Geometry check sheet. Reference: the model listing, model coordinates, mm. Face numbers are marked on the shaded views. Coordinates: 2 decimals unless noted, no trailing zeros. Loops run counter-clockwise (first coordinate to the right, second up) from the corner with the lowest first, then second, coordinate; pieces in that order, holes last. Notation, with made-up numbers: (51.25, 33) - (82.25, 33) arc R17 ccw to (82.25, 58) - close; hole circle Ø9 at (43, -14.75). An arc over 180 degrees is marked (long way). Write item = value, one per line. Start each with the question number.
from build123d import *

# Parameters (mm, degrees)
F0_W     = 200
F0_H     = 100
F1_DEPTH = 220
F2_T     = -12


with BuildPart() as f1:
    # F0 (on Front) → F1 (new body)
    with BuildSketch(Plane.XZ):
        Rectangle(F0_W, F0_H)
    extrude(amount=-F1_DEPTH)

    # F2
    f2_openings = [f1.faces().sort_by_distance(p)[0] for p in [
        (0, 0, 0),
    ]]
    offset(amount=F2_T, openings=f2_openings)


solid = f1.part
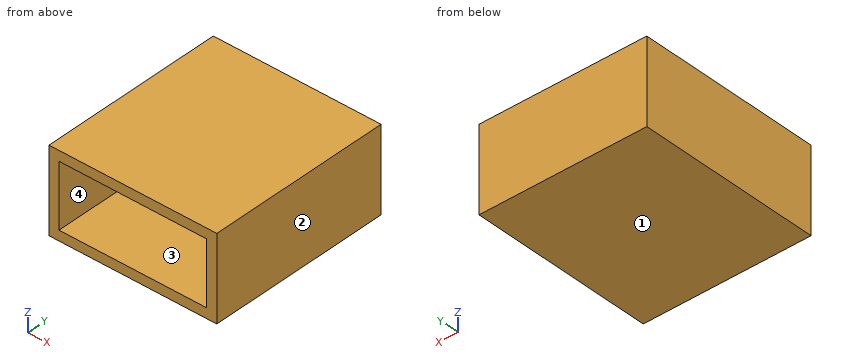
(1) Sectioned sample at C-C on y = 66. Enter the section's corners in (x, z).
(2) Depth check by flat-ended pin: pin 1 (12 mm diameter, centred on x = 73, z = 12, fed in from -Y). Enter the tip coordinate at first touch or a pass-through.
(3) Sectioned sample at A-A on x = -78. Enter the section's corners in (y, z).
(4) Scan lines: line 1 (X direction, y = 21, z = 15); line 2 (Z direction, x = -10.5, y = 177); line 3 (Y direction, x = 74, z = -29). Record each from-to range of solid material in increasing order.
(5) Sectioned sample at B-B on z = -30. Enter the section's corners in (x, y).
(6) Draft check along Z on the marked faces 1, 2, 3 and 4. Enter one of: pulls with the +Z half, pulls with the -Z half, needs draft (parallel to the pull), parting line crosses it, or undercut.
Working result:
q1.outline = (-100, -50) - (100, -50) - (100, 50) - (-100, 50) - close; hole (-88, -38) - (88, -38) - (88, 38) - (-88, 38) - close
q2.pin_1 = 208
q3.outline = (0, -50) - (220, -50) - (220, 50) - (0, 50) - (0, 38) - (208, 38) - (208, -38) - (0, -38) - close
q4.line_1 = -100 to -88, 88 to 100
q4.line_2 = -50 to -38, 38 to 50
q4.line_3 = 208 to 220
q5.outline = (-100, 0) - (-88, 0) - (-88, 208) - (88, 208) - (88, 0) - (100, 0) - (100, 220) - (-100, 220) - close
q6.face_1 = pulls with the -Z half
q6.face_2 = needs draft
q6.face_3 = undercut
q6.face_4 = undercut
